from build123d import *

# Parameters (mm, degrees)
CHAMFER1_SIZE       = 3.937
CHAMFER2_SIZE       = 2.54
SKETCH3_R           = 39.292876354
BOSS_EXTRUDE1_DEPTH = 13.15
SKETCH4_R           = 37.648699114
CUT_EXTRUDE1_DEPTH  = 2


with BuildPart() as part:
    # Sketch1 → Revolve1 (revolve)
    with BuildSketch(Plane(origin=(0, 0, 0), x_dir=(0, 0, -1), z_dir=(1, 0, 0))):
        Polygon((-107.78, -0.223974787), (-203.2, -0.223974787), (-203.2, 32.371025213), (-193.9, 32.371025213), (-193.9, 34.821025213), (-180.47, 34.821025213), (-180.47, 38.776025213), (-155.52, 38.776025213), (-155.52, 40.426025213), (-143.78, 41.376025213), (-143.78, 40.601025213), (-107.78, 40.601025213), align=None)
    revolve(axis=Axis((0, -0.223974787, 107.78), (0, 0, 1)))

    # Chamfer1
    chamfer1_edges = [part.edges().sort_by_distance(p)[0] for p in [
        (0, -39.223974787, 180.47),
    ]]
    chamfer(chamfer1_edges, length=CHAMFER1_SIZE)

    # Chamfer2
    # the kernel refuses this chamfer: 2.54 mm, written as the material it takes off along each edge
    with BuildSketch(Plane(origin=(0, -0.223974787, 193.9), x_dir=(0, 1, 0), z_dir=(1, 0, 0))) as chamfer2_piece_1_section:
        Polygon((35.045, -CHAMFER2_SIZE), (35.045 - CHAMFER2_SIZE, 0), (35.045, 0), align=None)
    chamfer2_piece_1 = revolve(axis=Axis((0, -0.223974787, 193.9), (0, 0, 1)), mode=Mode.PRIVATE)
    chamfer2_piece_1 = chamfer2_piece_1 - Plane(origin=(0, -0.223974787, 192.613574864), x_dir=(0, 1, 0), z_dir=(0, 0, -1)) * Cylinder(32.595, 141, mode=Mode.PRIVATE)
    add(chamfer2_piece_1, mode=Mode.SUBTRACT)

    # Sketch2 → Revolve2 (revolve)
    with BuildSketch(Plane(origin=(0, 0, 0), x_dir=(1, 0, 0), z_dir=(0, 1, 0))):
        Polygon((-40.825, -107.78), (-41.5, -107.78), (-41.5, -104.78), (-40.2, -104.78), (-40.2, -84.78), (-41.43, -84.78), (-41.43, -71.48), (-42, -71.48), (-42, -41.14), (-41.35, -41.14), (-41.35, -23.61), (-41.905, -23.61), (-41.905, -14.39), (-39.5, -5.13), (0, -5.13), (0, -107.78), align=None)
    revolve(axis=Axis((0, 0, 5.13), (0, 0, 1)))

    # Sketch3 → Boss-Extrude1 (add)
    with BuildSketch(Plane(origin=(0, 0, 5.13), x_dir=(-1, 0, 0), z_dir=(0, 0, -1))):
        Circle(SKETCH3_R)
    extrude(amount=BOSS_EXTRUDE1_DEPTH)

    # Sketch4 → Cut-Extrude1 (cut)
    with BuildSketch(Plane(origin=(0, 0, -8.02), x_dir=(-1, 0, 0), z_dir=(0, 0, -1))):
        Circle(SKETCH4_R)
    extrude(amount=-CUT_EXTRUDE1_DEPTH, mode=Mode.SUBTRACT)


solid = part.part
The listing builds one solid part. Answer for the finished solid, in the listing's coordinates (mm). A direction names the side the tool comes from. Give positions to 0.01 mm unless a question says otherwise; leave off trailing zeros. Write each loop counter-clockwise with the first axis right and the second up, starting at its lowest first coordinate (ties: lowest second). Pieces come first, ordered by that corner, then holes. Notation, with made-up numbers: (42.5, -3) -> (57.5, -3) arc R24 cw to (57.5, 31) -> close; hole circle Ø1 at (83.5, 52). An arc over 180 degrees is marked (long way). One line per question, with ' | ' between items. Start each with the question number.
1. Given pin 1 Ø3 at (y, z) = (24.5, 148.5) entering from +X; pin 2 Ø1 at (x, z) = (26.5, 178.5) entering from -Y; pin 3 Ø12 at (x, z) = (31.5, 15) entering from -Y, each flat-ended and moving along its own axis, determine where each tip first touches the part or whether it passes through.
2. Section A-A (z = 153) is taken. Determine the outline of the cut face in (x, y), plus the area to 3 significant figures.
3. For a pull along Z with two mould halves and no side action, classify faces 1 (the cylindrical face through (8.161, -36.753, -7.034)), 2 (the cylindrical face through (-39.584, -12.465, 106.259)), 3 (the conical face through (-10.606, 33.455, 180.224)), 4 (the flat face through (0, -38, -8.02)) as pulls with the +Z half, pulls with the -Z half, needs draft (parallel to the pull), parting line crosses it, or undercut.
4. For faces 5 (the cylindrical face through (27.484, 17.299, 198.439)), 6 (the flat face through (1, 1, -6.02)), 7 (the cylindrical face through (-38.344, -12.075, 94.64)), determine the directions among +Z, -Z, +X, -X, +Y, -Y from which every point of the face is accessible in a straight line to the end or side of a thin tool.
5. Find the intervals of material crossed by probe 1 along Y at (x, z) = (0, -7); probe 2 along Z at (x, y) = (-15.5, 4); probe 3 along Y at (x, z) = (-6, 21), in increasing order.
Response values:
1) pin 1: x = 34.06 | pin 2: y = -26.96 | pin 3: y = -33.25
2) outline: circle Ø81.71 at (0, -0.22) | area: 5,240 mm2
3) face 1: needs draft | face 2: undercut | face 3: pulls with the +Z half | face 4: pulls with the -Z half
4) face 5: +Z | face 6: -Z | face 7: none
5) probe 1: -39.29 to -37.65, 37.65 to 39.29 | probe 2: -6.02 to 203.2 | probe 3: -41.47 to 41.47
